from build123d import *

# Parameters (mm, degrees)
SKETCH2_R           = 3
BOSS_EXTRUDE1_DEPTH = 6
FILLET1_R           = 160
GROOVE_DEPTH        = 42.833001327
SKETCH5_W           = 6
SKETCH5_H           = 6
FINGERS_DEPTH       = 6
FILLET2_R           = 0.2


with BuildPart() as part:
    # Sketch2 → Boss-Extrude1 (new body)
    with BuildSketch(Plane.XY):
        with BuildLine():
            Line((0, 0), (-25, 0))
            Line((-25, 0), (-20.5, 25))
            ThreePointArc((-20.5, 25), (-12.5, 33), (-4.5, 25))
            Line((-4.5, 25), (0, 0))
        make_face()
        with Locations((-12.5, 25)):
            Circle(SKETCH2_R, mode=Mode.SUBTRACT)
    extrude(amount=BOSS_EXTRUDE1_DEPTH)

    # Fillet1
    fillet1_edges = [part.edges().sort_by_distance(p)[0] for p in [
        (-20.5, 25, 3),
        (-4.5, 25, 3),
    ]]
    fillet(fillet1_edges, radius=FILLET1_R)

    # Sketch4 → Groove (cut, through all)
    with BuildSketch(Plane.XY.offset(6)):
        with BuildLine():
            Line((-14, 0), (-14, 4.8))
            ThreePointArc((-14, 4.8), (-14.058578644, 4.941421356), (-14.2, 5))
            Line((-14.2, 5), (-15.8, 5))
            ThreePointArc((-15.8, 5), (-15.941421356, 5.058578644), (-16, 5.2))
            Line((-16, 5.2), (-16, 7.8))
            ThreePointArc((-16, 7.8), (-15.941421356, 7.941421356), (-15.8, 8))
            Line((-15.8, 8), (-14.2, 8))
            ThreePointArc((-14.2, 8), (-14.058578644, 8.058578644), (-14, 8.2))
            Line((-14, 8.2), (-14, 12))
            Line((-14, 12), (-11, 12))
            Line((-11, 12), (-11, 8.2))
            ThreePointArc((-11, 8.2), (-10.941421356, 8.058578644), (-10.8, 8))
            Line((-10.8, 8), (-9.2, 8))
            ThreePointArc((-9.2, 8), (-9.058578644, 7.941421356), (-9, 7.8))
            Line((-9, 7.8), (-9, 5.2))
            ThreePointArc((-9, 5.2), (-9.058578644, 5.058578644), (-9.2, 5))
            Line((-9.2, 5), (-10.8, 5))
            ThreePointArc((-10.8, 5), (-10.941421356, 4.941421356), (-11, 4.8))
            Line((-11, 4.8), (-11, 0))
            Line((-11, 0), (-14, 0))
        make_face()
    extrude(amount=-GROOVE_DEPTH, mode=Mode.SUBTRACT)

    # Sketch5 → Fingers (add)
    with BuildSketch(Plane.XZ):
        with Locations((-22, 3)):
            Rectangle(SKETCH5_W, SKETCH5_H)
        with Locations((-3, 3)):
            Rectangle(SKETCH5_W, SKETCH5_H)
    extrude(amount=FINGERS_DEPTH)

    # Fillet2
    fillet2_edges = [part.edges().sort_by_distance(p)[0] for p in [
        (-11, 0, 3),
        (-14, 0, 3),
    ]]
    fillet(fillet2_edges, radius=FILLET2_R)


solid = part.part
Design review of the part built by this model. Coordinates are the model's own, in mm. A direction names the side the tool comes from. Round coordinates to 2 decimals unless told otherwise and drop trailing zeros. Write each loop counter-clockwise with the first axis right and the second up, starting at its lowest first coordinate (ties: lowest second). Pieces come first, ordered by that corner, then holes. Notation, with made-up numbers: (-5.75, 19) - (43.25, 19) arc R29 cw to (43.25, 43) - close; hole circle Ø11 at (-7.5, -2.5). An arc over 180 degrees is marked (long way). Use a Markdown table: item, result. Add a question column.
1. We need section C-C (y = 17). State the section outline as (x, z) points, then the cut area to 3 significant figures.
2. For faces 1 (the face through (-9, 7, 3)), 2 (the face through (-11, 10, 3)), 3 (the face through (-4.11, 23, 3.04)), list the 3-axis set-ups (+Z, -Z, +X, -X, +Y, -Y) from which the entire face can be reached by the end or side of a thin tool; tool diameter is ignored.
3. Wall thickness on probe 1 along X at (y, z) = (9, 2.8); probe 2 along X at (y, z) = (6.5, 5.5); probe 3 along X at (y, z) = (18, 5.4): over which ranges is each line inside the solid? List them lowest first.
4. We need section B-B (y = 25). State the section outline as (x, z) points.
5. We need section A-A (x = -12.5). State the section outline as (y, z) points, then the cut area to 3 significant figures.
6. We need section D-D (x = -6.5). State the section outline as (y, z) points, then the cut area to 3 significant figures.
7. Clearance check with flat-ended pins moving along their axes: pin 1 (1.3 mm diameter, centred on x = -15, z = 2, fed in from +Y); pin 2 (1.4 mm diameter, centred on x = -9, z = 2, fed in from -Y); pin 3 (1.5 mm diameter, centred on x = -5, z = 4, fed in from +Y). State where each tip first meets the part, or that it passes through.
8. Mouldability with a two-part tool opening along Y and no side actions: class faces 4 (the face through (-16, 6, 3)), 5 (the face through (-11, 3, 3)), 6 (the face through (-23.227, 9.85, 2.958)) as +Y half, -Y half, draft (parallel to the pull), parting line (faces both ways), or undercut.
Output:
| question | item | result |
|---|---|---|
| 1 | outline | (-21.94, 0) - (-3.06, 0) - (-3.06, 6) - (-21.94, 6) - close |
| 1 | area | 113 mm2 |
| 2 | face 1 | +Z, -Z |
| 2 | face 2 | +Z, -Z, -Y |
| 2 | face 3 | +Z, -Z, +X, +Y |
| 3 | probe 1 | x = -23.38 to -14, -11 to -1.62 |
| 3 | probe 2 | x = -23.83 to -16, -9 to -1.17 |
| 3 | probe 3 | x = -21.76 to -3.24 |
| 4 | outline | (-20.58, 0) - (-15.5, 0) - (-15.5, 6) - (-20.58, 6) - close; (-9.5, 0) - (-4.42, 0) - (-4.42, 6) - (-9.5, 6) - close |
| 5 | outline | (12, 0) - (22, 0) - (22, 6) - (12, 6) - close; (28, 0) - (33, 0) - (33, 6) - (28, 6) - close |
| 5 | area | 90.0 mm2 |
| 6 | outline | (0, 0) - (30.29, 0) - (30.29, 6) - (0, 6) - close |
| 6 | area | 182 mm2 |
| 7 | pin 1 | stops at y = 32.78 |
| 7 | pin 2 | stops at y = 0 |
| 7 | pin 3 | stops at y = 29.29 |
| 8 | face 4 | undercut |
| 8 | face 5 | draft |
| 8 | face 6 | +Y half |
